from build123d import *

# Parameters (mm, degrees)
SKETCH1_W           = 25
SKETCH1_H           = 15
BOSS_EXTRUDE1_DEPTH = 2
CHAMFER1_SIZE       = 0.5
SKETCH2_R           = 1.5
BOSS_EXTRUDE2_DEPTH = 1
SKETCH3_W           = 3.5
SKETCH3_H           = 1.5
CUT_EXTRUDE1_DEPTH  = 1
CUT_EXTRUDE2_REACH  = 16.714
CUT_EXTRUDE3_REACH  = 16.714
FILLET2_R           = 0.875


with BuildPart() as part:
    # Sketch1 → Boss-Extrude1 (new body)
    with BuildSketch(Plane.XY):
        Rectangle(SKETCH1_W, SKETCH1_H)
    extrude(amount=BOSS_EXTRUDE1_DEPTH)

    # Chamfer1
    chamfer1_edges = [part.edges().sort_by_distance(p)[0] for p in [
        (-12.5, -7.5, 1),
        (12.5, -7.5, 1),
        (12.5, 7.5, 1),
        (-12.5, 7.5, 1),
    ]]
    chamfer(chamfer1_edges, length=CHAMFER1_SIZE)

    # Sketch2 → Boss-Extrude2 (add)
    with BuildSketch(Plane.XY.offset(2)):
        with Locations(Location((9.75, 4.7447, 0), (0, 0, 180))):
            Circle(SKETCH2_R)
    extrude(amount=BOSS_EXTRUDE2_DEPTH)

    # Sketch3 → Cut-Extrude1 (cut)
    with BuildSketch(Plane.XY.offset(2)):
        with Locations((-10, 4.7447)):
            Rectangle(SKETCH3_W, SKETCH3_H)
    extrude(amount=-CUT_EXTRUDE1_DEPTH, mode=Mode.SUBTRACT)

    # Sketch4 → Cut-Extrude2 (cut, up to next)
    with BuildSketch(Plane.XY.offset(2), mode=Mode.PRIVATE) as cut_extrude2_sk1:
        with BuildLine():
            Line((-11, -4.411618673), (0, -4.411618673))
            ThreePointArc((0, -4.411618673), (0.75, -5.161618673), (0, -5.911618673))
            Line((0, -5.911618673), (-11, -5.911618673))
            ThreePointArc((-11, -5.911618673), (-11.75, -5.161618673), (-11, -4.411618673))
        make_face()
    cut_extrude2_tool1 = extrude(cut_extrude2_sk1.sketch, amount=-CUT_EXTRUDE2_REACH, mode=Mode.PRIVATE) & part.part
    add(cut_extrude2_tool1.solids().sort_by_distance((-5.5, -5.161619, 2))[0], mode=Mode.SUBTRACT)

    # Sketch4<4> → Cut-Extrude3 (cut, up to next)
    with BuildSketch(Plane.XY.offset(2), mode=Mode.PRIVATE) as cut_extrude3_sk1:
        with BuildLine():
            Line((-11.75, -5.161618673), (-11.75, 0))
            ThreePointArc((-11.75, 0), (-11, 0.75), (-10.25, 0))
            Line((-10.25, 0), (-10.25, -5.161618673))
            ThreePointArc((-10.25, -5.161618673), (-11, -5.911618673), (-11.75, -5.161618673))
        make_face()
    cut_extrude3_tool1 = extrude(cut_extrude3_sk1.sketch, amount=-CUT_EXTRUDE3_REACH, mode=Mode.PRIVATE) & part.part
    add(cut_extrude3_tool1.solids().sort_by_distance((-11, -2.580809, 2))[0], mode=Mode.SUBTRACT)

    # Fillet2
    fillet2_edges = [part.edges().sort_by_distance(p)[0] for p in [
        (-10.25, -4.411618673, 1),
    ]]
    fillet(fillet2_edges, radius=FILLET2_R)


solid = part.part
Here's how the part is built. I have some questions about the finished solid (model axes, mm). A direction names the side the tool comes from. Round coordinates to 2 decimals unless told otherwise and drop trailing zeros. Write each loop counter-clockwise with the first axis right and the second up, starting at its lowest first coordinate (ties: lowest second). Pieces come first, ordered by that corner, then holes.
1. I need wall thicknesses on L1, parallel to Y at x = -9.25, z = 1.45; L2, parallel to X at y = -2.75, z = 0.4; L3, parallel to X at y = 5.25, z = 1.25. Which ranges of each line are inside material? Lowest first, please.
2. If we mould it in two halves opening along Y, with no side actions, what happens to faces 4 (the flat face through (-11.75, -3, 1)), 5 (the cylindrical face through (10.94, 5.66, 2.49)), 6 (the flat face through (0, 7.5, 1)), 7 (the flat face through (12.5, 0, 1))? For each: released by +Y, released by -Y, zero draft, split by the parting line, or undercut.
3. Suppose I cut it at A-A (x = -9). List the corners of the cut face in (y, z) for me.
4. Suppose I cut it at D-D (x = 5.5). List the corners of the cut face in (y, z) for me, and give its area (3 significant figures).
5. Suppose I cut it at B-B (y = -1). List the corners of the cut face in (x, z) for me.
6. Suppose I cut it at C-C (z = 0.7). List the corners of the cut face in (x, y) for me (3 decimals).
7. For faces 1 (the cylindrical face through (0.75, -5.15, 1.01)), 2 (the flat face through (-10, 5.495, 1.5)), 3 (the flat face through (10, 5, 3)), which set-ups out of +Z, -Z, +X, -X, +Y, -Y let a thin tool reach every point of the face, with its end or its side?
Answer sheet:
1. L1: y = -7.5 to -5.91, -4.41 to 3.99, 5.49 to 7.5
1. L2: x = -12.5 to -11.75, -10.25 to 12.5
1. L3: x = -12.5 to -11.75, -8.25 to 12.5
2. face 4: undercut
2. face 5: split by the parting line
2. face 6: released by +Y
2. face 7: zero draft
3. outline: (-7.5, 0) - (-5.91, 0) - (-5.91, 2) - (-7.5, 2) - close; (-4.41, 0) - (7.5, 0) - (7.5, 2) - (5.49, 2) - (5.49, 1) - (3.99, 1) - (3.99, 2) - (-4.41, 2) - close
4. outline: (-7.5, 0) - (7.5, 0) - (7.5, 2) - (-7.5, 2) - close
4. area: 30.0 mm2
5. outline: (-12.5, 0) - (-11.75, 0) - (-11.75, 2) - (-12.5, 2) - close; (-10.25, 0) - (12.5, 0) - (12.5, 2) - (-10.25, 2) - close
6. outline: (-12.5, -7) - (-12, -7.5) - (12, -7.5) - (12.5, -7) - (12.5, 7) - (12, 7.5) - (-12, 7.5) - (-12.5, 7) - close; hole (-11.75, -5.162) arc R0.75 ccw to (-11, -5.912) - (0, -5.912) arc R0.75 ccw to (0, -4.412) - (-9.375, -4.412) arc R0.875 cw to (-10.25, -3.537) - (-10.25, 0) arc R0.75 ccw to (-11.75, 0) - close
7. face 1: +Z, -Z
7. face 2: +Z
7. face 3: +Z, +X, -X, +Y, -Y
